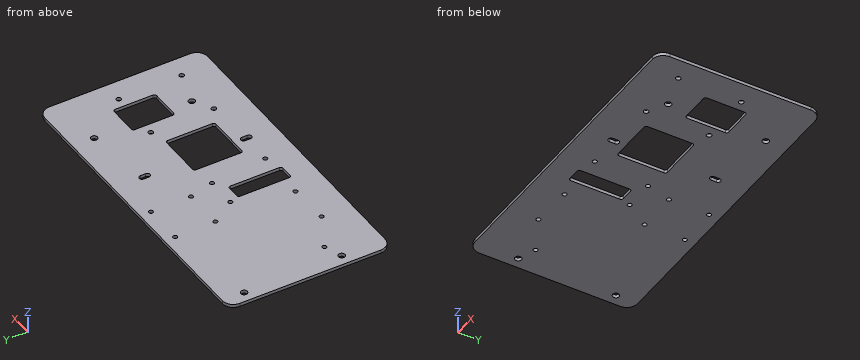
from build123d import *

# Parameters (mm, degrees)
SKETCH_1_W          = 290
SKETCH_1_H          = 150
SKETCH_1_R          = 2.25
SKETCH_1_R_2        = 2
EXTRUDE_1_DEPTH     = 3
SKETCH_5_R          = 3
CUT_EXTRUDE_1_DEPTH = 10
SKETCH_6_W          = 29.947475637
SKETCH_6_H          = 39.048227512
SKETCH_6_W_2        = 43.213980646
SKETCH_6_H_2        = 45.404503952
SKETCH_6_W_3        = 14.915916247
SKETCH_6_H_3        = 49.22754674
CUT_EXTRUDE_2_DEPTH = 10
FILLET_1_R          = 2
FILLET_2_R          = 10


with BuildPart() as part:
    # 스케치1 → 보스-돌출1 (new body)
    with BuildSketch(Plane.XY):
        Rectangle(SKETCH_1_W, SKETCH_1_H)
        with Locations((76.027180087, 13)):
            Circle(SKETCH_1_R, mode=Mode.SUBTRACT)
        with Locations((76.027180087, -45)):
            Circle(SKETCH_1_R, mode=Mode.SUBTRACT)
        with Locations((125.027180087, -45)):
            Circle(SKETCH_1_R, mode=Mode.SUBTRACT)
        with Locations((125.027180087, 13)):
            Circle(SKETCH_1_R, mode=Mode.SUBTRACT)
        with Locations((-118.572819913, -29)):
            Circle(SKETCH_1_R_2, mode=Mode.SUBTRACT)
        with Locations((-84.572819913, -47)):
            Circle(SKETCH_1_R_2, mode=Mode.SUBTRACT)
        with Locations((1.027180087, -46.9)):
            Circle(SKETCH_1_R_2, mode=Mode.SUBTRACT)
        with Locations((-3.672819913, 5)):
            Circle(SKETCH_1_R_2, mode=Mode.SUBTRACT)
        with Locations((-31.572819913, 5)):
            Circle(SKETCH_1_R_2, mode=Mode.SUBTRACT)
        with Locations((-46.772819913, -45.8)):
            Circle(SKETCH_1_R_2, mode=Mode.SUBTRACT)
        with Locations((-9.772819913, 28)):
            Circle(SKETCH_1_R_2, mode=Mode.SUBTRACT)
        with Locations((-46.772819913, 28)):
            Circle(SKETCH_1_R_2, mode=Mode.SUBTRACT)
        with Locations((-46.772819913, 65)):
            Circle(SKETCH_1_R_2, mode=Mode.SUBTRACT)
        with Locations((-9.772819913, 65)):
            Circle(SKETCH_1_R_2, mode=Mode.SUBTRACT)
        with BuildLine():
            Line((28.527180087, 43.5), (28.527180087, 48.5))
            ThreePointArc((28.527180087, 48.5), (31.027180087, 51), (33.527180087, 48.5))
            Line((33.527180087, 48.5), (33.527180087, 43.5))
            ThreePointArc((33.527180087, 43.5), (31.027180087, 41), (28.527180087, 43.5))
        make_face(mode=Mode.SUBTRACT)
        with BuildLine():
            Line((33.527180087, -45), (33.527180087, -50))
            ThreePointArc((33.527180087, -50), (31.027180087, -52.5), (28.527180087, -50))
            Line((28.527180087, -50), (28.527180087, -45))
            ThreePointArc((28.527180087, -45), (31.027180087, -42.5), (33.527180087, -45))
        make_face(mode=Mode.SUBTRACT)
    extrude(amount=-EXTRUDE_1_DEPTH)

    # 스케치5 → 컷-돌출1 (cut)
    with BuildSketch(Plane.XY):
        with Locations((-135, 55)):
            Circle(SKETCH_5_R)
        with Locations((-135, -35)):
            Circle(SKETCH_5_R)
        with Locations((93, 55)):
            Circle(SKETCH_5_R)
        with Locations((93, -35)):
            Circle(SKETCH_5_R)
    extrude(amount=-CUT_EXTRUDE_1_DEPTH, mode=Mode.SUBTRACT)

    # 스케치6 → 컷-돌출2 (cut)
    with BuildSketch(Plane.XY):
        with Locations((100.550839394, 4.607183656)):
            Rectangle(SKETCH_6_W, SKETCH_6_H)
        with Locations((38.78961529, -13.625434023)):
            Rectangle(SKETCH_6_W_2, SKETCH_6_H_2)
        with Locations((-21.905088543, -28.00761485)):
            Rectangle(SKETCH_6_W_3, SKETCH_6_H_3)
    extrude(amount=-CUT_EXTRUDE_2_DEPTH, mode=Mode.SUBTRACT)

    # 필렛1
    fillet_1_edges = [part.edges().sort_by_distance(p)[0] for p in [
        (85.577101575, -14.9169301, -1.5),
        (85.577101575, 24.131297412, -1.5),
        (115.524577212, 24.131297412, -1.5),
        (115.524577212, -14.9169301, -1.5),
        (17.182624967, -36.327685999, -1.5),
        (17.182624967, 9.076817953, -1.5),
        (60.396605613, 9.076817953, -1.5),
        (60.396605613, -36.327685999, -1.5),
        (-29.363046666, -52.62138822, -1.5),
        (-29.363046666, -3.39384148, -1.5),
        (-14.447130419, -3.39384148, -1.5),
        (-14.447130419, -52.62138822, -1.5),
    ]]
    fillet(fillet_1_edges, radius=FILLET_1_R)

    # 필렛2
    fillet_2_edges = [part.edges().sort_by_distance(p)[0] for p in [
        (-145, 75, -1.5),
        (145, 75, -1.5),
        (145, -75, -1.5),
        (-145, -75, -1.5),
    ]]
    fillet(fillet_2_edges, radius=FILLET_2_R)


solid = part.part
The listing builds one solid part. Answer for the finished solid, in the listing's coordinates (mm). Give positions to 0.01 mm unless a question says otherwise; leave off trailing zeros. Write each loop counter-clockwise with the first axis right and the second up, starting at its lowest first coordinate (ties: lowest second). Pieces come first, ordered by that corner, then holes.
Item 1: Section C-C, the plane z = -2.45 is taken. Count the separate pieces of the cut face and the enclosed holes in it, plus the area to 3 significant figures.
Item 2: Flat-ended cylindrical pins translate along their axes: P1, Ø6.5, axis at x = -9.77, y = 65, coming from the +Z side; P2, Ø3, axis at x = -46.77, y = 65, coming from the -Z side. Find the tip coordinate at first contact, or state that the pin passes through.
Item 3: Section A-A, the plane y = -19 is taken. Write down the section's boundary in (x, z).
Item 4: Find the intervals of material crossed by line 1 along X through (y, z) = (-23.5, -0.15); line 2 along Y through (x, z) = (93, -1.3); line 3 along X through (y, z) = (1, -2), in increasing order.
Item 5: Section B-B, the plane x = 109 is taken. Write down the section's boundary in (y, z), plus the area to 3 significant figures.
Completed:
1. separate pieces: 1
1. enclosed holes: 23
1. area: 39,200 mm2
2. P1: stops at z = 0
2. P2: passes through
3. outline: (-145, -3) - (-29.36, -3) - (-29.36, 0) - (-145, 0) - close; (-14.45, -3) - (17.18, -3) - (17.18, 0) - (-14.45, 0) - close; (60.4, -3) - (145, -3) - (145, 0) - (60.4, 0) - close
4. line 1: x = -145 to -29.36, -14.45 to 17.18, 60.4 to 145
4. line 2: y = -75 to -38, -32 to -14.92, 24.13 to 52, 58 to 75
4. line 3: x = -145 to 17.18, 60.4 to 85.58, 115.52 to 145
5. outline: (-75, -3) - (-14.92, -3) - (-14.92, 0) - (-75, 0) - close; (24.13, -3) - (75, -3) - (75, 0) - (24.13, 0) - close
5. area: 333 mm2
